Check sheet for the modelled part. Datum: model origin and axes. Units: mm. Face numbers are marked on the shaded views. A direction names the side the tool comes from. Give positions to 0.01 mm unless a question says otherwise; leave off trailing zeros. Order: outer loops, then holes, each group sorted by start corner. A loop starts at its lowest first (then second) coordinate and runs counter-clockwise, first axis right, second up.
```python
from build123d import *

# Parameters (mm, degrees)
BOSS_EXTRUDE1_DEPTH = 4
SKETCH3_W           = 6
SKETCH3_H           = 8
CUT_EXTRUDE1_DEPTH  = 15
FILLET1_R           = 4
SKETCH4_R           = 1.25
CUT_EXTRUDE2_DEPTH  = 23.090722034
FILLET2_R           = 5
FILLET3_R           = 5
SKETCH6_R           = 1.45
CUT_EXTRUDE3_DEPTH  = 28.202941017


with BuildPart() as part:
    # Sketch1 → Boss-Extrude1 (new, symmetric)
    with BuildSketch(Plane.XY):
        Polygon((15, 5), (15, -5), (5, -5), (-5, -10), (-18, -10), (-18, -5), (-5, -5), (-5, 5), (-18, 5), (-18, 10), (-5, 10), (5, 5), align=None)
    extrude(amount=BOSS_EXTRUDE1_DEPTH, both=True)

    # Sketch3 → Cut-Extrude1 (cut)
    with BuildSketch(Plane(origin=(15, 0, 0), x_dir=(0, 0, -1), z_dir=(1, 0, 0))):
        with Locations((-1, 0)):
            Rectangle(SKETCH3_W, SKETCH3_H)
    extrude(amount=-CUT_EXTRUDE1_DEPTH, mode=Mode.SUBTRACT)

    # Fillet1
    fillet1_edges = [part.edges().sort_by_distance(p)[0] for p in [
        (0, -4, 1),
        (0, 4, 1),
    ]]
    fillet(fillet1_edges, radius=FILLET1_R - 0.0001)  # a hair under: the kernel refuses the full size

    # Sketch4 → Cut-Extrude2 (cut, through all)
    with BuildSketch(Plane(origin=(0, 0, -4), x_dir=(-1, 0, 0), z_dir=(0, 0, -1))):
        with Locations((-4, 0)):
            Circle(SKETCH4_R)
        with Locations((-8, 0)):
            Circle(SKETCH4_R)
    extrude(amount=-CUT_EXTRUDE2_DEPTH, mode=Mode.SUBTRACT)

    # Fillet2
    fillet2_edges = [part.edges().sort_by_distance(p)[0] for p in [
        (-5, 5, 0),
        (-5, -5, 0),
    ]]
    fillet(fillet2_edges, radius=FILLET2_R - 0.0001)  # a hair under: the kernel refuses the full size

    # Fillet3
    fillet3_edges = [part.edges().sort_by_distance(p)[0] for p in [
        (-5, 10, 0),
        (5, 5, 0),
        (5, -5, 0),
        (-5, -10, 0),
    ]]
    fillet(fillet3_edges, radius=FILLET3_R)

    # Sketch6 → Cut-Extrude3 (cut, through all)
    with BuildSketch(Plane(origin=(0, 10, 0), x_dir=(1, 0, 0), z_dir=(0, 1, 0))):
        with Locations(Location((-14, 0, 0), (0, 0, 180))):
            Circle(SKETCH6_R)
    extrude(amount=-CUT_EXTRUDE3_DEPTH, mode=Mode.SUBTRACT)


solid = part.part
```
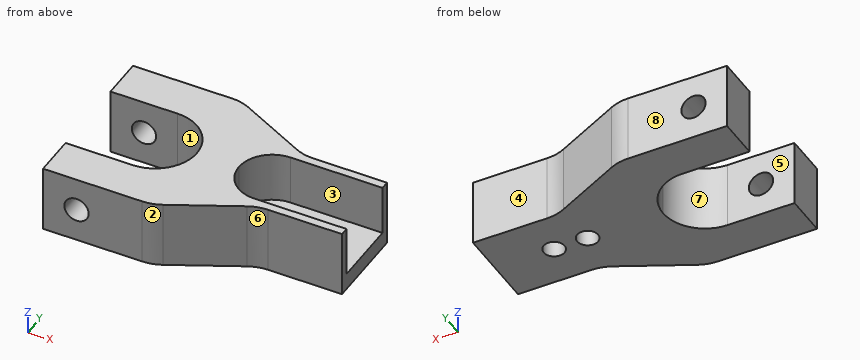
(1) Thickness scan on L1, parallel to Z at x = -14, y = -7.2; L2, parallel to Y at x = 9.5, z = 1.25; L3, parallel to Y at x = 8, z = -2.5. Record the ranges inside material, lowest first.
(2) Sectioned sample at B-B (z = -3.25). Count the separate pieces of the cut face and the enclosed holes in it, plus the area to 3 significant figures.
(3) Sectioned sample at A-A (x = 8). Enter the section's corners in (y, z).
(4) Go/stop test with flat-tipped pins: P1, Ø3, axis at x = 4, y = 0, coming from the +Z side; P2, Ø3, axis at x = 9, z = 0.5, coming from the +Y side; P3, Ø2, axis at x = 3.5, y = 7.5, coming from the +Z side; P4, Ø4, axis at x = 11.5, z = -1.5, coming from the -Y side. Record where each tip stops, or that it passes through.
(5) Release check for a two-part mould opening along Y. For the marked faces 5, 6, 7 and 8 record: released by +Y, released by -Y, zero draft, split by the parting line, or undercut.
(6) Sectioned sample at C-C (x = -14). Enter the section's corners in (y, z), plus the area to 3 significant figures.
(7) Tool access check on the marked faces 1, 2, 3 and 4. Record the directions out of +Z, -Z, +X, -X, +Y, -Y that give a thin tool (end or side, any length) a straight path to the whole face; none if there is none.
Values follow:
1. L1: z = -4 to -1.45, 1.45 to 4
1. L2: y = -5 to -4, 4 to 5
1. L3: y = -5 to -1.25, 1.25 to 5
2. separate pieces: 1
2. enclosed holes: 2
2. area: 381 mm2
3. outline: (-5, -4) - (-1.25, -4) - (-1.25, -2) - (-4, -2) - (-4, 4) - (-5, 4) - close; (1.25, -4) - (5, -4) - (5, 4) - (4, 4) - (4, -2) - (1.25, -2) - close
4. P1: stops at z = -2
4. P2: stops at y = 5
4. P3: passes through
4. P4: stops at y = -5
5. face 5: undercut
5. face 6: released by -Y
5. face 7: undercut
5. face 8: released by +Y
6. outline: (-10, -4) - (-5, -4) - (-5, -1.45) - (-10, -1.45) - close; (-10, 1.45) - (-5, 1.45) - (-5, 4) - (-10, 4) - close; (5, -4) - (10, -4) - (10, -1.45) - (5, -1.45) - close; (5, 1.45) - (10, 1.45) - (10, 4) - (5, 4) - close
6. area: 51.0 mm2
7. face 1: +Z, -Z, -X
7. face 2: +Z, -Z, +X, -Y
7. face 3: +Z, +X
7. face 4: +Z, -Z, +X, +Y
